Can you work these out from the model? Positions are in its coordinate system, mm. A direction names the side the tool comes from. Round coordinates to 2 decimals unless told otherwise and drop trailing zeros. Order: outer loops, then holes, each group sorted by start corner. A loop starts at its lowest first (then second) coordinate and runs counter-clockwise, first axis right, second up. Notation, with made-up numbers: M -1.75,62 L 6.25,62 A27 cw 6.25,101 Z; hole C 79,-31 d7. An arc over 180 degrees is marked long. Answer as a JSON object with one key per item and string values. Group by question number.
from build123d import *

# Parameters (mm, degrees)
F0_W     = 139.4626796246
F0_H     = 10.6887500733
F1_DEPTH = 38.1
F2_W     = 139.4626796246
F2_H     = 10.6887500733
F3_DEPTH = 38.1
F4_W     = 11.3281075606
F4_H     = 76.2
F5_DEPTH = 25.4
F6_W     = 11.3281150824
F6_H     = 76.2
F7_DEPTH = 25.4
F8_W     = 81.4380571246
F8_H     = 41.2280112505
F9_DEPTH = 15.24


# Not quite as in the source:
# - the program builds the solid bodies; features that only make, move or delete a surface that nothing else refers to are left out


with BuildPart() as f1:
    # F0 (on Front) → F1 (new body)
    with BuildSketch(Plane.XZ):
        Rectangle(F0_W, F0_H)
    extrude(amount=F1_DEPTH)

    # F2 (on face) → F3 (join)
    with BuildSketch(Plane(origin=(0, 0, 0), x_dir=(-1, 0, 0), z_dir=(0, 1, 0))):
        Rectangle(F2_W, F2_H)
    extrude(amount=F3_DEPTH)

    # F4 (on face) → F5 (join)
    with BuildSketch(Plane(origin=(0, 0, -5.3443750367), x_dir=(1, 0, 0), z_dir=(0, 0, -1))):
        with Locations((-47.5903637707, 0)):
            Rectangle(F4_W, F4_H)
    extrude(amount=F5_DEPTH)

    # F6 (on face) → F7 (join)
    with BuildSketch(Plane(origin=(0, 0, -5.3443750367), x_dir=(1, 0, 0), z_dir=(0, 0, -1))):
        with Locations((41.6097603738, 0)):
            Rectangle(F6_W, F6_H)
    extrude(amount=F7_DEPTH)

    # F8 (on face) → F9 (join)
    with BuildSketch(Plane.XY.offset(5.3443750367)):
        with Locations((-24.4314149022, 0)):
            Rectangle(F8_W, F8_H)
    extrude(amount=F9_DEPTH)


solid = f1.part
Item 1: Suppose I cut it at B-B, the plane y = 26.5. Write out the boundary of the cut face in (x, z).
Item 2: On a 3-axis mill with a long thin cutter (end or side, diameter ignored), from which of +Z, -Z, +X, -X, +Y, -Y can I reach the whole of each face in a straight line? I mean faces 1 (the face through (16.288, 0, 13)), 2 (the face through (-53.254, 1, -18)), 3 (the face through (-2, -1, -5.344)), 4 (the face through (59, -1, -5.344)). Say none if no direction works.
Item 3: Suppose I cut it at D-D, the plane z = 12. Write out the boundary of the cut face in (x, y), and give its area (3 significant figures).
Item 4: Suppose I cut it at A-A, the plane z = -7.5. Write out the boundary of the cut face in (x, y).
Item 5: Suppose I cut it at C-C, the plane x = -50.5. Write out the boundary of the cut face in (y, z).
Item 6: If we mould it in two halves opening along X, with no side actions, what happens to faces 5 (the face through (-65.15, 0, 13)), 6 (the face through (-41.926, 1, -18)), 7 (the face through (-48, -1, -30.744))? For each: +X half, -X half, draft (parallel to the pull), parting line (faces both ways), or undercut.
Item 7: I need wall thicknesses on line 1 (X direction, y = 15, z = -16); line 2 (Z direction, x = 16, y = -30.5); line 3 (Y direction, x = -29, z = 11.5). Which ranges of each line are inside material? Lowest first, please.
Item 8: I'm going to push flat-ended pins straight in: pin 1 Ø4.5 at (x, z) = (-18.5, 10) entering from -Y; pin 2 Ø1.5 at (y, z) = (-11.5, -11) entering from +X; pin 3 Ø20.5 at (y, z) = (10.5, -16.5) entering from -X. Where does each tip first touch, or does it pass through?
Computed:
{
 "1": {"outline": "M -69.73,-5.34 L -53.25,-5.34 L -53.25,-30.74 L -41.93,-30.74 L -41.93,-5.34 L 35.95,-5.34 L 35.95,-30.74 L 47.27,-30.74 L 47.27,-5.34 L 69.73,-5.34 L 69.73,5.34 L -69.73,5.34 Z"},
 "2": {"face 1": "+Z, +X, +Y, -Y", "face 2": "-Z, -X, +Y, -Y", "face 3": "-Z, +Y, -Y", "face 4": "-Z, +X, +Y, -Y"},
 "3": {"outline": "M -65.15,-20.61 L 16.29,-20.61 L 16.29,20.61 L -65.15,20.61 Z", "area": "3,360 mm^2"},
 "4": {"outline": "M -53.25,-38.1 L -41.93,-38.1 L -41.93,38.1 L -53.25,38.1 Z; M 35.95,-38.1 L 47.27,-38.1 L 47.27,38.1 L 35.95,38.1 Z"},
 "5": {"outline": "M -38.1,-30.74 L 38.1,-30.74 L 38.1,5.34 L 20.61,5.34 L 20.61,20.58 L -20.61,20.58 L -20.61,5.34 L -38.1,5.34 Z"},
 "6": {"face 5": "-X half", "face 6": "undercut", "face 7": "draft"},
 "7": {"line 1": "x = -53.25 to -41.93, 35.95 to 47.27", "line 2": "z = -5.34 to 5.34", "line 3": "y = -20.61 to 20.61"},
 "8": {"pin 1": "stops at y = -20.61", "pin 2": "stops at x = 47.27", "pin 3": "stops at x = -53.25"}
}
